from build123d import *

# Parameters (mm, degrees)
BOSS_EXTRUDE2_DEPTH            = 30
BOSS_EXTRUDE2_DEPTH_BACK       = 30
EXTRUDE_THIN2_DEPTH            = 25
EXTRUDE_THIN2_DEPTH_BACK       = 25
SKETCH2_W                      = 60
SKETCH2_H                      = 5
BOSS_EXTRUDE3_DEPTH            = 100
BOSS_EXTRUDE4_DEPTH            = 30
BOSS_EXTRUDE4_DEPTH_BACK       = 30
CUT_EXTRUDE2_REACH             = 143.361
SKETCH4_W                      = 60
SKETCH4_H                      = 5
CUT_EXTRUDE2_DIRECTION_2_REACH = 143.361
BOSS_EXTRUDE5_DEPTH            = 30
BOSS_EXTRUDE5_DEPTH_BACK       = 30
DRONE_ARM_FIT_CUT_DEPTH        = 50
CUT_EXTRUDE3_START             = -60
SKETCH8_W                      = 5
SKETCH8_H                      = 5
CUT_EXTRUDE3_DEPTH             = 60


with BuildPart() as part:
    # Sketch1 → Boss-Extrude2 (new, two sides: drawn at the far end of the back side and taken through both)
    with BuildSketch(Plane.XY.offset(-BOSS_EXTRUDE2_DEPTH_BACK)):
        Polygon((-13.01396445, -23.830717844), (0, -23.830717844), (0, -18.830717844), (-11.698214449, -18.830717844), (-50, 2.827283512), (-50, 13.432214294), (-55, 13.432214294), (-55, -0.089432632), align=None)
        Polygon((0, -18.830717844), (0, -23.830717844), (13.01396445, -23.830717844), (55, -0.089432632), (55, 13.432214294), (50, 13.432214294), (50, 2.827283512), (11.698214449, -18.830717844), align=None)
        with BuildLine():
            Line((-11.698214449, -18.830717844), (0, -18.830717844))
            Line((0, -18.830717844), (0, -8))
            ThreePointArc((0, -8), (-8, 0), (0, 8))
            Line((0, 8), (0, 13.432214294))
            Line((0, 13.432214294), (-50, 13.432214294))
            Line((-50, 13.432214294), (-50, 2.827283512))
            Line((-50, 2.827283512), (-11.698214449, -18.830717844))
        make_face()
        with BuildLine():
            Line((0, -8), (0, -18.830717844))
            Line((0, -18.830717844), (11.698214449, -18.830717844))
            Line((11.698214449, -18.830717844), (50, 2.827283512))
            Line((50, 2.827283512), (50, 13.432214294))
            Line((50, 13.432214294), (0, 13.432214294))
            Line((0, 13.432214294), (0, 8))
            ThreePointArc((0, 8), (5.656854249, 5.656854249), (8, 0))
            ThreePointArc((8, 0), (5.656854249, -5.656854249), (0, -8))
        make_face()
    extrude(amount=BOSS_EXTRUDE2_DEPTH + BOSS_EXTRUDE2_DEPTH_BACK)

    # Sketch1<5> → Extrude-Thin2 (add, two sides: drawn at the far end of the back side and taken through both)
    with BuildSketch(Plane.XY.offset(-EXTRUDE_THIN2_DEPTH_BACK)):
        Polygon((50, 13.432214294), (50, 38.432214294), (50, 63.432214294), (-50, 63.432214294), (-50, 38.432214294), (-50, 13.432214294), (-55, 13.432214294), (-55, 38.432214294), (-55, 68.432214294), (55, 68.432214294), (55, 38.432214294), (55, 13.432214294), align=None)
    extrude(amount=EXTRUDE_THIN2_DEPTH + EXTRUDE_THIN2_DEPTH_BACK)

    # Sketch2 → Boss-Extrude3 (add)
    with BuildSketch(Plane.ZY.offset(-50)):
        with Locations((0, 37.694873029)):
            Rectangle(SKETCH2_W, SKETCH2_H)
    extrude(amount=BOSS_EXTRUDE3_DEPTH)

    # Sketch1<6> → Boss-Extrude4 (add, two sides: drawn at the far end of the back side and taken through both)
    with BuildSketch(Plane.XY.offset(-BOSS_EXTRUDE4_DEPTH_BACK)):
        Polygon((-55, -0.089432632), (-55, 13.432214294), (-70, 13.432214294), (-70, -8.839581066), (-16.961214453, -38.830717844), (16.961214453, -38.830717844), (70, -8.839581066), (70, 13.432214294), (55, 13.432214294), (55, -0.089432632), (13.01396445, -23.830717844), (-13.01396445, -23.830717844), align=None)
    extrude(amount=BOSS_EXTRUDE4_DEPTH + BOSS_EXTRUDE4_DEPTH_BACK)

    # Cut-Extrude2: up to this face of the body (flat: up to its plane)
    cut_extrude2_end = Plane(part.part.faces().sort_by_distance((-55, 40.932214294, 0))[0])
    # Sketch4 → Cut-Extrude2 (cut, up to the picked face)
    with BuildSketch(Plane(origin=(-50, 0, 0), x_dir=(0, 0, -1), z_dir=(1, 0, 0)), mode=Mode.PRIVATE) as cut_extrude2_sk1:
        with Locations((0, 65.932214294)):
            Rectangle(SKETCH4_W, SKETCH4_H)
    cut_extrude2_tool1 = split(extrude(cut_extrude2_sk1.sketch, amount=-CUT_EXTRUDE2_REACH, mode=Mode.PRIVATE), bisect_by=cut_extrude2_end, keep=Keep.BOTH, mode=Mode.PRIVATE)
    add(cut_extrude2_tool1.solids().sort_by(Axis((-50, 65.932214, 0), (-1, 0, 0)))[0], mode=Mode.SUBTRACT)

    # Cut-Extrude2 direction 2: up to this face of the body (flat: up to its plane)
    cut_extrude2_direction_2_end = Plane(part.part.faces().sort_by_distance((55, 40.932214294, 0))[0])
    # Sketch4 → Cut-Extrude2 direction 2 (cut, up to the picked face)
    with BuildSketch(Plane(origin=(-50, 0, 0), x_dir=(0, 0, -1), z_dir=(1, 0, 0)), mode=Mode.PRIVATE) as cut_extrude2_direction_2_sk1:
        with Locations((0, 65.932214294)):
            Rectangle(SKETCH4_W, SKETCH4_H)
    cut_extrude2_direction_2_tool1 = split(extrude(cut_extrude2_direction_2_sk1.sketch, amount=CUT_EXTRUDE2_DIRECTION_2_REACH, mode=Mode.PRIVATE), bisect_by=cut_extrude2_direction_2_end, keep=Keep.BOTH, mode=Mode.PRIVATE)
    add(cut_extrude2_direction_2_tool1.solids().sort_by(Axis((-50, 65.932214, 0), (1, 0, 0)))[0], mode=Mode.SUBTRACT)

    # Sketch1<7> → Boss-Extrude5 (add, two sides: drawn at the far end of the back side and taken through both)
    with BuildSketch(Plane.XY.offset(-BOSS_EXTRUDE5_DEPTH_BACK)):
        Polygon((-70, 13.432214294), (-55, 13.432214294), (-50, 13.432214294), (-50, 38.432214294), (-50, 63.432214294), (-70, 63.432214294), (-70, 38.432214294), align=None)
        Polygon((50, 38.432214294), (50, 13.432214294), (55, 13.432214294), (70, 13.432214294), (70, 38.432214294), (70, 63.432214294), (50, 63.432214294), align=None)
    extrude(amount=BOSS_EXTRUDE5_DEPTH + BOSS_EXTRUDE5_DEPTH_BACK)

    # Sketch7 → Drone Arm fit cut (cut)
    with BuildSketch(Plane(origin=(0, 63.432214294, 0), x_dir=(1, 0, 0), z_dir=(0, 1, 0))):
        Polygon((-70, -12.5), (-70, 12.5), (-65, 12.5), (-65, 7.5), (-60, 7.5), (-60, 12.5), (-60, 17.5), (-55, 17.5), (-55, -17.5), (-60, -17.5), (-60, -12.5), (-60, -7.5), (-65, -7.5), (-65, -12.5), align=None)
    drone_arm_fit_cut = extrude(amount=-DRONE_ARM_FIT_CUT_DEPTH, mode=Mode.SUBTRACT)

    # Mirror Drone arm fit cut: Drone Arm fit cut across plane
    add(drone_arm_fit_cut.mirror(Plane(origin=(0, 0, 0), x_dir=(0, 0, 1), z_dir=(1, 0, 0))), mode=Mode.SUBTRACT)

    # Sketch8 → Cut-Extrude3 (cut)
    with BuildSketch(Plane.XY.offset(30).offset(CUT_EXTRUDE3_START)):
        with Locations((-60, 50.932214294)):
            Rectangle(SKETCH8_W, SKETCH8_H)
        with Locations((-60, 30.932214294)):
            Rectangle(SKETCH8_W, SKETCH8_H)
    cut_extrude3 = extrude(amount=CUT_EXTRUDE3_DEPTH, mode=Mode.SUBTRACT)

    # Mirror1: Cut-Extrude3 across plane
    add(cut_extrude3.mirror(Plane(origin=(0, 0, 0), x_dir=(0, 0, 1), z_dir=(1, 0, 0))), mode=Mode.SUBTRACT)


solid = part.part
Geometry: final body of the model. Coordinates: model frame, mm. A direction names the side the tool comes from. Give positions to 0.01 mm unless a question says otherwise; leave off trailing zeros. Write each loop counter-clockwise with the first axis right and the second up, starting at its lowest first coordinate (ties: lowest second). Pieces come first, ordered by that corner, then holes. Notation, with made-up numbers: (26, 4.25) -> (43, 4.25) arc R19 ccw to (43, 41.25) -> close; hole circle Ø2 at (67.5, 14.5). An arc over 180 degrees is marked (long way). Answer as a JSON object with one key per item and string values.
1. Cut plane C-C on z = 26.5. Count the separate pieces of the cut face and the enclosed holes in it, and give its area (3 significant figures).
Ans:
{"separate pieces": "1", "enclosed holes": "6", "area": "7,930 mm^2"}
2. Cut plane B-B on z = 5. Output: boundary loops of the cut face in (x, y).
Ans:
{"outline": "(-70, -8.84) -> (-16.96, -38.83) -> (16.96, -38.83) -> (70, -8.84) -> (70, 13.43) -> (55, 13.43) -> (55, 63.43) -> (50, 63.43) -> (50, 40.19) -> (-50, 40.19) -> (-50, 63.43) -> (-55, 63.43) -> (-55, 13.43) -> (-70, 13.43) -> close; hole (-50, 13.43) -> (50, 13.43) -> (50, 35.19) -> (-50, 35.19) -> close; hole circle Ø16 at (0, 0)"}
3. Cut plane D-D on y = -5. Output: boundary loops of the cut face in (x, z) (3 decimals).
Ans:
{"outline": "(-70, -30) -> (-6.245, -30) -> (-6.245, 30) -> (-70, 30) -> close; (6.245, -30) -> (70, -30) -> (70, 30) -> (6.245, 30) -> close"}
4. Mould query, pull axis Z, two halves, no side actions, for faces 4 (the flat face through (1, 12, 30)), 5 (the flat face through (-61, 53.432, 21)), 6 (the flat face through (63, 39, -7.5)), 7 (the flat face through (-60, 21, -13)). Classes: pulls with the +Z half, pulls with the -Z half, needs draft (parallel to the pull), parting line crosses it, or undercut.
Ans:
{"face 4": "pulls with the +Z half", "face 5": "needs draft", "face 6": "undercut", "face 7": "undercut"}
5. Access query for faces 1 (the flat face through (-61, 28.432, -21)), 2 (the flat face through (-58, 39, -17.5)), 3 (the flat face through (70, 11, 0)). Directions: +Z, -Z, +X, -X, +Y, -Y. A direction counts if a zero-diameter tool reaches every point of the face in a straight line with its end or side. Return the directions, or none.
Ans:
{"face 1": "+Z, -Z", "face 2": "+Y", "face 3": "+Z, -Z, +X, +Y, -Y"}
6. Ray query, probe 1 along X at (y, z) = (26.5, -8.5); probe 2 along X at (y, z) = (53, -19); probe 3 along Y at (x, z) = (-7, 6). Return the intervals inside material, ascending. Write a range as from..to.
Ans:
{"probe 1": "x = -65..-60, -55..-50, 50..55, 60..65", "probe 2": "x = -70..-62.5, -57.5..-50, 50..57.5, 62.5..70", "probe 3": "y = -38.83..-3.87, 3.87..13.43, 35.19..40.19"}
7. Contact query for flat-ended pins moving along their axis: pin 1 (6 mm diameter, centred on x = -30, z = 20, fed in from -Y); pin 2 (8 mm diameter, centred on x = -32, z = -13.5, fed in from +Y); pin 3 (10 mm diameter, centred on x = 25, z = -8, fed in from -Y). Output: stop coordinate, or through.
Ans:
{"pin 1": "stops at y = -33.15", "pin 2": "stops at y = 40.19", "pin 3": "stops at y = -37.11"}
